Here's how the part is built. I have some questions about the finished solid (model axes, mm). Face numbers are marked on the shaded views. A direction names the side the tool comes from. Give positions to 0.01 mm unless a question says otherwise; leave off trailing zeros. Loops run counter-clockwise (first coordinate to the right, second up) from the corner with the lowest first, then second, coordinate; pieces in that order, holes last. Notation, with made-up numbers: (16, -23) - (54, -23) arc R18 cw to (54, -17) - close; hole circle Ø1 at (60.25, 76.5). An arc over 180 degrees is marked (long way). Put each result on its own line as item: value. Start each with the question number.
Autodesk Fusion 360 part; units mm, degrees
sketch "Sketch1" plane through (0, 0, 0) normal (0, 0, 1) x (1, 0, 0)
  circle A0 centre (0, 0) radius 47.225
  circle A1 centre (0, 0) radius 57.5
  circle A2 centre (0, 52) radius 1.7
  circle A3 centre (0, -52) radius 1.7
  circle A4 centre (-52, 0) radius 1.7
  circle A5 centre (52, 0) radius 1.7
  dimension "d1" = 94.45
  dimension "d2" = 115
  dimension "d3" = 3.4
  dimension "d4" = 3.4
  dimension "d5" = 3.4
  dimension "d6" = 3.4
extrude "Extrude4" add sketch "Sketch1" along normal blind 3.1 contours A2 | A3 | A4 | A5 makes body 1 at (53.6979, -0.0847, 2.0667) makes body 2 at (-50.3021, -0.0847, 2.0667) makes body 3 at (-1.5975, 52.5814, 2.0667) makes body 4 at (-1.5975, -51.4186, 2.0667)
extrude "Extrude5" add sketch "Sketch1" along normal blind 13 bodies 1 2 3 4
extrude "Extrude6" add sketch "Sketch1" along normal blind 3 contours A0 bodies 1
sketch "Sketch2" plane through (0, 0, 13) normal (0, 0, 1) x (-1, 0, 0)
  circle A0 centre (0, -52) radius 1.7
  circle A1 centre (52, 0) radius 1.7
  circle A2 centre (0, 52) radius 1.7
  circle A3 centre (-52, 0) radius 1.7
  circle A4 centre (0, 0) radius 47.225
  circle A5 centre (0, 0) radius 57.5
  line L0 (-15, -35) -> (-34, -35)
  line L1 (-34, -35) -> (-34, -57)
  line L2 (-34, -57) -> (-15, -57)
  line L3 (-15, -57) -> (-15, -35)
  line L4 (-34, -35) -> (-15, -35)
  line L5 (-15, -35) -> (-15, -31)
  line L6 (-15, -31) -> (-34, -31)
  line L7 (-34, -31) -> (-34, -35)
extrude "Extrude7" cut sketch "Sketch2" against normal blind 7.5 contours A4 L0 L4 L7 | A4 A5 L0 L1 L3 L4 bodies 1
extrude "Extrude3" [suppressed]
extrude "Extrude2" [suppressed]
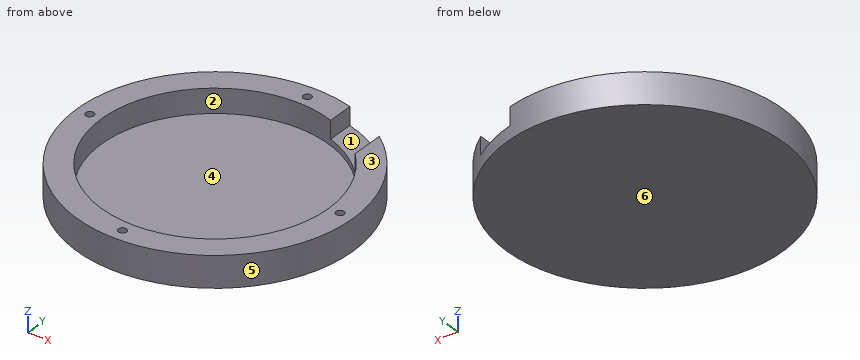
1) Which directions (+Z, -Z, +X, -X, +Y, -Y) give clear straight access to the entire face, cutting with the end or side of a thin tool? Please do the marked faces 1, 2 and 3.
2) Suppose I cut it at A-A on x = 0. Please give me the cut outline in (y, z) (3 decimals), plus the area to 3 significant figures.
3) I need wall thicknesses on line 1 (Y direction, x = 0, z = 10.5) (3 decimals); line 2 (X direction, y = 0.5, z = 10.75); line 3 (X direction, y = -4, z = 7). Which ranges of each line are inside material? Lowest first, please.
4) I'm going to push flat-ended pins straight in: P1, Ø5.5, axis at x = 0, y = 52, coming from the -Z side; P2, Ø6, axis at y = 48, z = 8, coming from the +X side; P3, Ø12, axis at x = -34, y = 11, coming from the +Z side; P4, Ø2, axis at y = 43, z = 7.5, coming from the +X side. Where does each tip first touch, or does it pass through?
5) Suppose I cut it at B-B on z = 7.5. Please give me the cut outline in (x, y) (3 decimals).
6) Thinking about a two-plate mould opening in Y: for the marked faces 4, 5 and 6, which applies, pulls with the +Y half, pulls with the -Y half, needs draft (parallel to the pull), parting line crosses it, or undercut?
7) Suppose I cut it at D-D on x = 27. Please give me the cut outline in (y, z).
Ans:
1. face 1: +Z, +Y
1. face 2: +Z
1. face 3: +Z, +X, -X, +Y, -Y
2. outline: (-57.5, 0) - (57.5, 0) - (57.5, 13) - (53.7, 13) - (53.7, 3.1) - (50.3, 3.1) - (50.3, 13) - (47.225, 13) - (47.225, 3) - (-47.225, 3) - (-47.225, 13) - (-50.3, 13) - (-50.3, 3.1) - (-53.7, 3.1) - (-53.7, 13) - (-57.5, 13) - close
2. area: 483 mm²
3. line 1: y = -57.5 to -53.7, -50.3 to -47.225, 47.225 to 50.3, 53.7 to 57.5
3. line 2: x = -57.5 to -53.62, -50.38 to -47.22, 47.22 to 50.38, 53.62 to 57.5
3. line 3: x = -57.36 to -47.06, 47.06 to 57.36
4. P1: stops at z = 0
4. P2: stops at x = 35.79
4. P3: stops at z = 3
4. P4: stops at x = 39.27
5. outline: (15, 44.779) - (15, 55.509) arc R57.5 ccw (long way) to (34, 46.371) - (34, 32.775) arc R47.225 cw (long way) to start; hole circle Ø3.4 at (-52, 0); hole circle Ø3.4 at (0, -52); hole circle Ø3.4 at (0, 52); hole circle Ø3.4 at (52, 0)
6. face 4: undercut
6. face 5: parting line crosses it
6. face 6: needs draft
7. outline: (-50.77, 0) - (50.77, 0) - (50.77, 5.5) - (38.75, 5.5) - (38.75, 3) - (-38.75, 3) - (-38.75, 13) - (-50.77, 13) - close
